Part model, mm, in its own coordinate system. A direction names the side the tool comes from. Coordinates: 2 decimals unless noted, no trailing zeros. Order: outer loops, then holes, each group sorted by start corner. A loop starts at its lowest first (then second) coordinate and runs counter-clockwise, first axis right, second up. Notation, with made-up numbers: (37.25, 13) - (85.25, 13) arc R16 cw to (85.25, 22) - close; hole circle Ø9 at (86.5, 42). An arc over 180 degrees is marked (long way). Use a Markdown table: item, result. Add a question column.
1) Wall check: L1, parallel to X at y = -9.75, z = 17; L2, parallel to Z at x = -10, y = -11. Give the ranges that are in metal, low to high. Write a range as [from, to].
2) Two-plate mould, pull along Z, no slides. Class faces 1 (the face through (0, -10, -60)), 2 (the face through (0, -10, 55)), 3 (the face through (-27, 0, 5)): +Z half, -Z half, draft (parallel to the pull), parting line (faces both ways), or undercut.
3) Saw through at B-B on x = -7.5. List the corners of the cut face in (y, z).
4) Saw through at A-A on z = -35. List the corners of the cut face in (x, y).
5) Saw through at C-C on y = -15.5. List the corners of the cut face in (x, z).
6) Tool access for faces 4 (the face through (-25, -10, -1)), 5 (the face through (30, -10, -1)): list every direction of +Z, -Z, +X, -X, +Y, -Y with a clear straight run to the whole face (end or side of a thin tool).
```python
from build123d import *

# Parameters (mm, degrees)
F2_DEPTH = 20


with BuildPart() as f2:
    # F0 (on Front) → F2 (new body)
    with BuildSketch(Plane.XZ):
        Polygon((-25, 0), (-30, 0), (-30, -60), (0, -60), (0, -55.198602), (-25, -55.198602), align=None)
        Polygon((0, 55), (0, 60), (-30, 60), (-30, 0), (-25, 0), (-25, 55), align=None)
        Polygon((30, 60), (0, 60), (0, 55), (25, 55), (25, 0), (30, 0), align=None)
        Polygon((30, -60), (30, 0), (25, 0), (25, -55.198602), (0, -55.198602), (0, -60), align=None)
    extrude(amount=F2_DEPTH)


solid = f2.part
```
Results are:
| question | item | result |
|---|---|---|
| 1 | L1 | [-30, -25], [25, 30] |
| 1 | L2 | [-60, -55.2], [55, 60] |
| 2 | face 1 | -Z half |
| 2 | face 2 | undercut |
| 2 | face 3 | draft |
| 3 | outline | (-20, -60) - (0, -60) - (0, -55.2) - (-20, -55.2) - close; (-20, 55) - (0, 55) - (0, 60) - (-20, 60) - close |
| 4 | outline | (-30, -20) - (-25, -20) - (-25, 0) - (-30, 0) - close; (25, -20) - (30, -20) - (30, 0) - (25, 0) - close |
| 5 | outline | (-30, -60) - (30, -60) - (30, 60) - (-30, 60) - close; hole (-25, -55.2) - (25, -55.2) - (25, 55) - (-25, 55) - close |
| 6 | face 4 | +Y, -Y |
| 6 | face 5 | +Z, -Z, +X, +Y, -Y |
